Could you check a few things on this model? Use its own coordinates, in mm. Face numbers are marked on the shaded views. A direction names the side the tool comes from. Coordinates: 2 decimals unless noted, no trailing zeros. Order: outer loops, then holes, each group sorted by start corner. A loop starts at its lowest first (then second) coordinate and runs counter-clockwise, first axis right, second up. Notation, with made-up numbers: M -7,7 L 0,7 A21 ccw 0,18 Z; hole C -8,26 d9. An arc over 180 degrees is marked long. One line per question, with ' | ' between items. Start each with the question number.
from build123d import *

# Parameters (mm, degrees)
SKETCH1_W           = 245.429281818
SKETCH1_H           = 117.865734126
BOSS_EXTRUDE1_DEPTH = 86.36
CHAMFER1_SIZE       = 16.18000066
SKETCH2_R           = 39.915781682
BOSS_EXTRUDE2_DEPTH = 148.082


with BuildPart() as part:
    # Sketch1 → Boss-Extrude1 (new body)
    with BuildSketch(Plane(origin=(0, 0, 0), x_dir=(1, 0, 0), z_dir=(0, 1, 0))):
        Rectangle(SKETCH1_W, SKETCH1_H)
    extrude(amount=BOSS_EXTRUDE1_DEPTH)

    # Chamfer1
    chamfer1_edges = [part.edges().sort_by_distance(p)[0] for p in [
        (0, 86.36, 58.932867063),
        (0, 0, 58.932867063),
        (-122.714640909, 43.18, 58.932867063),
    ]]
    chamfer(chamfer1_edges, length=CHAMFER1_SIZE)

    # Sketch2 → Boss-Extrude2 (add)
    with BuildSketch(Plane(origin=(0, 86.36, 0), x_dir=(1, 0, 0), z_dir=(0, 1, 0))):
        with Locations(Location((0, 0, 0), (0, 0, 270))):
            Circle(SKETCH2_R)
    extrude(amount=BOSS_EXTRUDE2_DEPTH)


solid = part.part
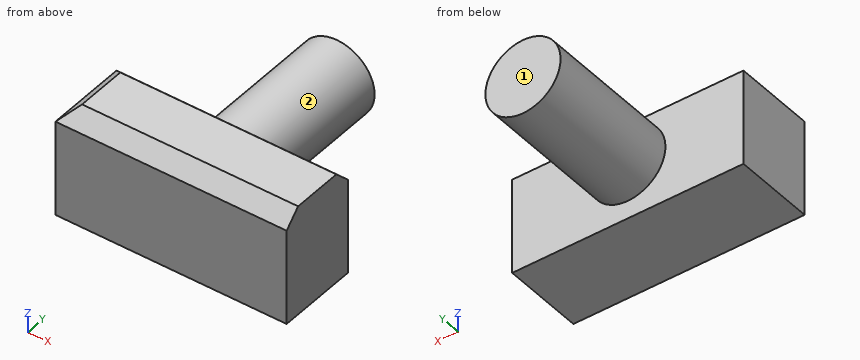
(1) Imagine slicing it at D-D, the plane x = 0. Write out the boundary of the cut face in (y, z).
(2) Imagine slicing it at A-A, the plane x = -47. Write out the boundary of the cut face in (y, z).
(3) Imagine slicing it at B-B, the plane z = 0. Write out the boundary of the cut face in (x, y), plus the area to 3 significant figures.
(4) On a 3-axis mill with a long thin cutter (end or side, diameter ignored), from which of +Z, -Z, +X, -X, +Y, -Y can I reach the whole of each face in a straight line? I mean the marked faces 1 and 2. Say none if no direction works.
(5) If I drill on line 1 along Z through (x, y) = (-1, 217); line 2 along Y through (x, z) = (41, -2); line 3 along X through (y, z) = (205, 17), over which ranges is the centre line in solid material (lowest first)? Write a range as from..to.
(6) Imagine slicing it at C-C, the plane y = 133. Write out the boundary of the cut face in (x, z).
(7) For P1, Ø1.5, axis at x = 55, z = 26.5, coming from the +Y side; P2, Ø5, axis at y = 131, z = 8, coming from the +X side; P3, Ø3, axis at y = 112.5, z = -34, coming from the +X side, each with a flat end and sliding along its axis, tell me the tip position at first contact or that it passes through.
Answers:
1) outline: M 0,-58.93 L 86.36,-58.93 L 86.36,-39.92 L 234.44,-39.92 L 234.44,39.92 L 86.36,39.92 L 86.36,42.75 L 70.18,58.93 L 16.18,58.93 L 0,42.75 Z
2) outline: M 0,-58.93 L 86.36,-58.93 L 86.36,42.75 L 70.18,58.93 L 16.18,58.93 L 0,42.75 Z
3) outline: M -122.71,0 L 122.71,0 L 122.71,86.36 L 39.92,86.36 L 39.92,234.44 L -39.92,234.44 L -39.92,86.36 L -122.71,86.36 Z | area: 33,000 mm²
4) face 1: +Z, -Z, +X, -X, +Y | face 2: +Y
5) line 1: -39.9..39.9 | line 2: 0..86.36 | line 3: -36.11..36.11
6) outline: C 0,0 d79.83
7) P1: y = 86.36 | P2: x = 39.54 | P3: x = 23.17
